Source: three-view drawing plus pictorial views. Frame: mm from the lowest corner of the part. Give positions to 0.01 mm unless a question says otherwise; leave off trailing zeros. Write each loop counter-clockwise with the first axis right and the second up, starting at its lowest first coordinate (ties: lowest second). Pieces come first, ordered by that corner, then holes.
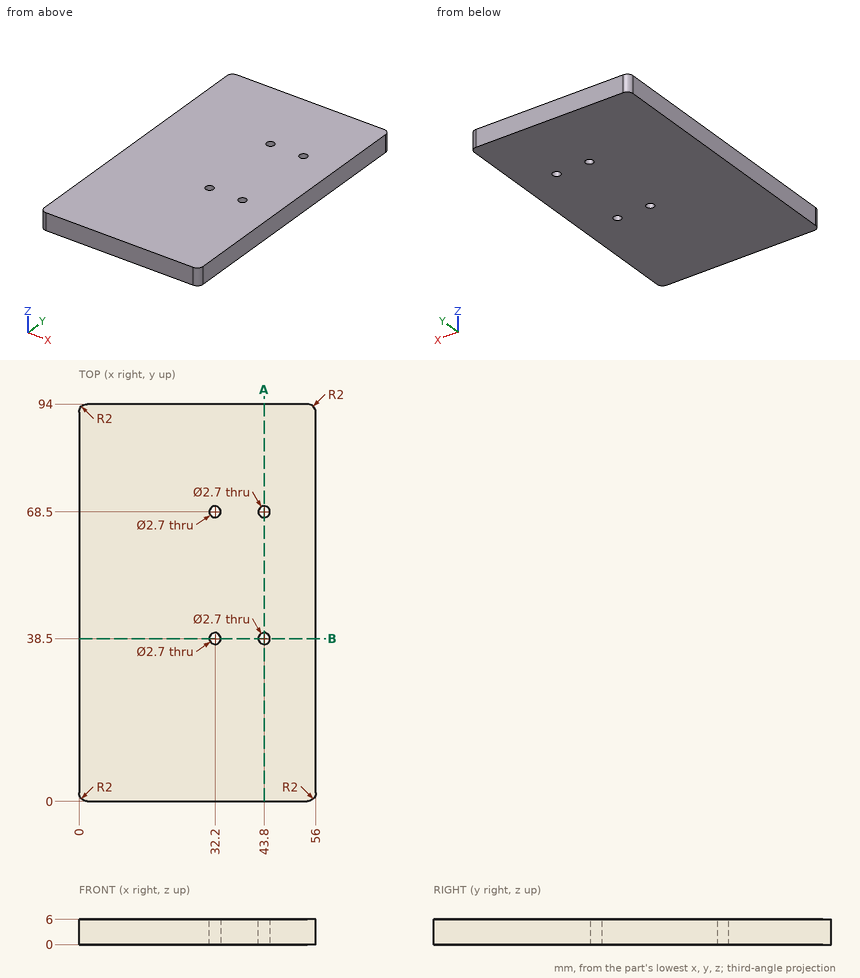
Q1. Section A-A on x = 43.8. Output: boundary loops of the cut face in (y, z).
Filled sheet:
outline: (0, 0) - (37.15, 0) - (37.15, 6) - (0, 6) - close; (39.85, 0) - (67.15, 0) - (67.15, 6) - (39.85, 6) - close; (69.85, 0) - (94, 0) - (94, 6) - (69.85, 6) - close
Q2. Section B-B on y = 38.5. Output: boundary loops of the cut face in (x, z).
Filled sheet:
outline: (0, 0) - (30.85, 0) - (30.85, 6) - (0, 6) - close; (33.55, 0) - (42.45, 0) - (42.45, 6) - (33.55, 6) - close; (45.15, 0) - (56, 0) - (56, 6) - (45.15, 6) - close
Q3. Pin query (flat end, axial travel): P1, Ø4.5, axis at x = 32.2, y = 68.5, coming from the +Z side; P2, Ø2, axis at x = 32.2, y = 38.5, coming from the -Z side. Return the tip coordinate at first contact, or that it passes through.
Filled sheet:
P1: stops at z = 6
P2: passes through
Q4. Ray query, line 1 along Y through (x, z) = (32.2, 4.7); line 2 along X through (y, z) = (68.5, 2.7). Return the intervals inside material, ascending.
Filled sheet:
line 1: y = 0 to 37.15, 39.85 to 67.15, 69.85 to 94
line 2: x = 0 to 30.85, 33.55 to 42.45, 45.15 to 56
